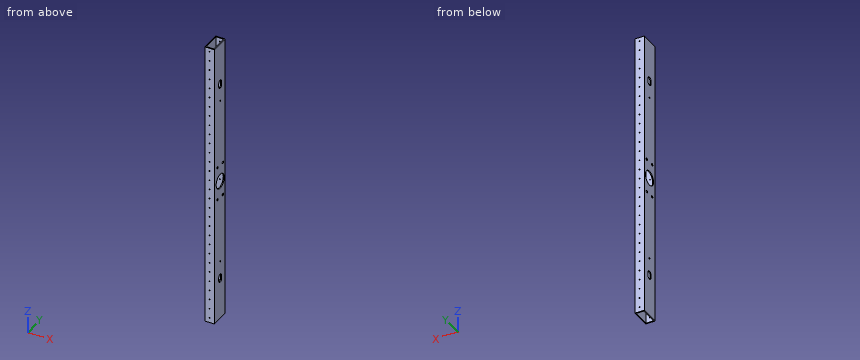
```python
from build123d import *

# Parameters (mm, degrees)
SKETCH1_W           = 25.4
SKETCH1_H           = 50.8
SKETCH1_W_2         = 20.32
SKETCH1_H_2         = 45.72
EXTRUDE_THIN1_DEPTH = 379.4125
SKETCH2_R           = 1.27
CUT_EXTRUDE1_DEPTH  = 384.008844749
LPATTERN1_COUNT     = 30
LPATTERN1_PITCH     = 25.4
SKETCH4_R           = 19.05
SKETCH4_R_2         = 1.9304
CUT_EXTRUDE2_DEPTH  = 382.109124997
SKETCH5_R           = 3.175
CUT_EXTRUDE3_DEPTH  = 382.109124997


with BuildPart() as part:
    # Sketch1 → Extrude-Thin1 (new, symmetric)
    with BuildSketch(Plane.XY):
        Rectangle(SKETCH1_W, SKETCH1_H)
        Rectangle(SKETCH1_W_2, SKETCH1_H_2, mode=Mode.SUBTRACT)
    extrude(amount=EXTRUDE_THIN1_DEPTH, both=True)

    # Sketch2 → Cut-Extrude1 (cut, through all)
    with BuildSketch(Plane(origin=(0, 25.4, 0), x_dir=(1, 0, 0), z_dir=(0, 1, 0))):
        with Locations(Location((0, 366.7125, 0), (0, 0, 270))):
            Circle(SKETCH2_R)
    cut_extrude1 = extrude(amount=-CUT_EXTRUDE1_DEPTH, mode=Mode.SUBTRACT)

    # LPattern1: Cut-Extrude1 ×30
    with Locations(*[(0, 0, i * LPATTERN1_PITCH) for i in range(1, LPATTERN1_COUNT)]):
        add(cut_extrude1, mode=Mode.SUBTRACT)

    # Sketch4 → Cut-Extrude2 (cut, through all)
    with BuildSketch(Plane.ZY.offset(12.7)):
        with Locations((0, 1.651)):
            Circle(SKETCH4_R)
        with Locations((-222.25, 1.651)):
            Circle(SKETCH4_R_2)
        with Locations((222.25, 1.651)):
            Circle(SKETCH4_R_2)
        with BuildLine():
            Line((263.906, 8.509), (272.796, 8.509))
            ThreePointArc((272.796, 8.509), (279.654, 1.651), (272.796, -5.207))
            Line((272.796, -5.207), (263.906, -5.207))
            ThreePointArc((263.906, -5.207), (257.048, 1.651), (263.906, 8.509))
        make_face()
        with BuildLine():
            Line((-263.906, 8.509), (-272.796, 8.509))
            ThreePointArc((-272.796, 8.509), (-279.654, 1.651), (-272.796, -5.207))
            Line((-272.796, -5.207), (-263.906, -5.207))
            ThreePointArc((-263.906, -5.207), (-257.048, 1.651), (-263.906, 8.509))
        make_face()
    extrude(amount=-CUT_EXTRUDE2_DEPTH, mode=Mode.SUBTRACT)

    # Sketch5 → Cut-Extrude3 (cut, through all)
    with BuildSketch(Plane.ZY.offset(12.7)):
        with Locations((-44.45, 14.351)):
            Circle(SKETCH5_R)
        with Locations((-44.45, -11.049)):
            Circle(SKETCH5_R)
        with Locations((44.45, 14.351)):
            Circle(SKETCH5_R)
        with Locations((44.45, -11.049)):
            Circle(SKETCH5_R)
    extrude(amount=-CUT_EXTRUDE3_DEPTH, mode=Mode.SUBTRACT)


solid = part.part
```
Here's how the part is built. I have some questions about the finished solid (model axes, mm). Round coordinates to 2 decimals unless told otherwise and drop trailing zeros. Order: outer loops, then holes, each group sorted by start corner. A loop starts at its lowest first (then second) coordinate and runs counter-clockwise, first axis right, second up. Notation, with made-up numbers: M -1,-9.75 L 10,-9.75 A21 cw 10,-3.75 Z; hole C -10.75,-3.5 d2. An arc over 180 degrees is marked long. Use CSV: the item, a comma, the result in double quotes.
1) I want a section at A-A (z = 0). List the corners of the cut face in (x, y) for me.
Taken from the geometry:
outline,"M -12.7,-25.4 L 12.7,-25.4 L 12.7,-17.4 L 10.16,-17.4 L 10.16,-22.86 L -10.16,-22.86 L -10.16,-17.4 L -12.7,-17.4 Z; M -12.7,20.7 L -10.16,20.7 L -10.16,22.86 L 10.16,22.86 L 10.16,20.7 L 12.7,20.7 L 12.7,25.4 L -12.7,25.4 Z"
2) I want a section at B-B (z = 302.5). List the corners of the cut face in (x, y) for me.
Taken from the geometry:
outline,"M -12.7,-25.4 L 12.7,-25.4 L 12.7,25.4 L -12.7,25.4 Z; hole M -10.16,-22.86 L 10.16,-22.86 L 10.16,22.86 L -10.16,22.86 Z"
3) I need wall thicknesses on line 1 along Y through (x, z) = (7.5, -9); line 2 along X through (y, z) = (3.5, -189); line 3 along Y through (x, z) = (11.5, 44.45). Which ranges of each line are inside material? Lowest first, please. Write a range as [from, to].
Taken from the geometry:
line 1,"[-25.4, -22.86], [22.86, 25.4]"
line 2,"[-12.7, -10.16], [10.16, 12.7]"
line 3,"[-25.4, -14.22], [-7.87, 11.18], [17.53, 25.4]"
